Input: part model. Units: mm. Frame: model coordinates. A direction names the side the tool comes from. Coordinates: 2 decimals unless noted, no trailing zeros. Write each loop counter-clockwise with the first axis right and the second up, starting at its lowest first coordinate (ties: lowest second). Pieces come first, ordered by that corner, then holes. Notation, with made-up numbers: (23, -10.5) -> (70, -10.5) arc R14 cw to (70, -1.5) -> close; hole circle Ø1 at (-0.5, 84). An arc over 180 degrees is marked (long way). Use one line per item in the form item = value. Start each with the question number.
(1) First-contact query: pin 1 (5.5 mm diameter, centred on x = 8.31, z = 83.82, fed in from +Y); pin 2 (1.2 mm diameter, centred on x = -1, y = -1, fed in from +Z); pin 3 (1.9 mm diameter, centred on y = 1, z = 79, fed in from +X); pin 4 (2 mm diameter, centred on y = -1, z = 7.5, fed in from +X). Flat tips, straight axial feed; report the tip coordinate or a pass-through.
(2) Cut plane A-A on z = 0. Return the cut outline in (x, y) (3 decimals).
(3) Cut plane C-C on y = 2. Return the cut outline in (x, z) (3 decimals), plus the area to 3 significant figures.
(4) Ray query, line 1 along X through (y, z) = (1.25, 83.82); line 2 along X through (y, z) = (0, 0); line 3 along Z through (x, y) = (60, 1.75). Return the intervals inside material, ascending.
(5) Cut plane D-D on x = -28.5. Return the cut outline in (y, z) (3 decimals).
(6) Set-up query: faces 5 (the face through (-12.7, 0, 79)), 6 (the face through (12.7, 0, 79)), 7 (the face through (0, -2, 77.47)). Return all of +Z, -Z, +X, -X, +Y, -Y with unobstructed straight access to the full face (end or side cutting, diameter ignored); none if empty.
(7) Cut plane B-B on x = 0. Return the cut outline in (y, z) (3 decimals), plus the area to 3 significant figures.
(8) Pull-direction query (Z, two-part tool) for faces 1 (the face through (8.45, 0.04, 80.65)), 2 (the face through (20.6, -0.044, 65.413)), 3 (the face through (0.09, 0.89, 83.27)), 4 (the face through (0.1, 1.5, 88.9)); classes: released by +Z, released by -Z, zero draft, split by the parting line, or undercut.
```python
from build123d import *

# Parameters (mm, degrees)
SKETCH1_R                   = 76.2
SKETCH1_R_2                 = 68.58
BOSS_EXTRUDE1_DEPTH         = 3.175
BOSS_EXTRUDE2_DEPTH         = 6.35
FILLET1_R                   = 6.35
CUT_EXTRUDE1_DEPTH          = 11.43
F_3_8_0_25_DIAMETER_HOLE2_D = 6.35


with BuildPart() as part:
    # Sketch1 → Boss-Extrude1 (new, symmetric)
    with BuildSketch(Plane(origin=(0, 0, 0), x_dir=(1, 0, 0), z_dir=(0, 1, 0))):
        with Locations(Location((0, 0, 0), (0, 0, 270))):
            Circle(SKETCH1_R)
        with Locations(Location((0, 0, 0), (0, 0, 270))):
            Circle(SKETCH1_R_2, mode=Mode.SUBTRACT)
    extrude(amount=BOSS_EXTRUDE1_DEPTH, both=True)

    # Sketch2 → Boss-Extrude2 (add)
    with BuildSketch(Plane(origin=(0, 3.175, 0), x_dir=(1, 0, 0), z_dir=(0, 1, 0))):
        with BuildLine():
            Line((-12.7, -88.9), (-12.7, -75.134213245))
            ThreePointArc((-12.7, -75.134213245), (0, -76.2), (12.7, -75.134213245))
            Line((12.7, -75.134213245), (12.7, -88.9))
            Line((12.7, -88.9), (-12.7, -88.9))
        make_face()
    extrude(amount=-BOSS_EXTRUDE2_DEPTH)

    # Fillet1
    fillet1_edges = [part.edges().sort_by_distance(p)[0] for p in [
        (12.7, 0, 88.9),
        (-12.7, 0, 88.9),
    ]]
    fillet(fillet1_edges, radius=FILLET1_R)

    # Sketch3 → Cut-Extrude1 (cut)
    with BuildSketch(Plane.XY.offset(88.9)):
        with BuildLine():
            Line((-4.064, -3.175), (4.064, -3.175))
            ThreePointArc((4.064, -3.175), (0, 0.889), (-4.064, -3.175))
        make_face()
    extrude(amount=-CUT_EXTRUDE1_DEPTH, mode=Mode.SUBTRACT)

    # 3/8 (0.25) Diameter Hole2 (through all)
    with Locations(Plane(origin=(-8.3058, -3.175, 83.82), x_dir=(0, 0, -1), z_dir=(0, -1, 0))):
        with Locations((0, 0), (0, 16.6116)):
            Hole(F_3_8_0_25_DIAMETER_HOLE2_D / 2)


solid = part.part
```
Values:
q1.pin_1 = through
q1.pin_2 = 77.47
q1.pin_3 = 12.7
q1.pin_4 = 75.92
q2.outline = (-76.2, -3.175) -> (-68.58, -3.175) -> (-68.58, 3.175) -> (-76.2, 3.175) -> close; (68.58, -3.175) -> (76.2, -3.175) -> (76.2, 3.175) -> (68.58, 3.175) -> close
q3.outline = (-12.7, 75.134) arc R76.2 ccw (long way) to (12.7, 75.134) -> (12.7, 82.55) arc R6.35 ccw to (6.35, 88.9) -> (-6.35, 88.9) arc R6.35 ccw to (-12.7, 82.55) -> close; hole circle Ø137.16 at (0, 0); hole circle Ø6.35 at (-8.306, 83.82); hole circle Ø6.35 at (8.306, 83.82)
q3.area = 3,720 mm2
q4.line_1 = -12.57 to -11.48, -5.13 to 5.13, 11.48 to 12.57
q4.line_2 = -76.2 to -68.58, 68.58 to 76.2
q4.line_3 = -46.97 to -33.21, 33.21 to 46.97
q5.outline = (-3.175, -70.67) -> (3.175, -70.67) -> (3.175, -62.378) -> (-3.175, -62.378) -> close; (-3.175, 62.378) -> (3.175, 62.378) -> (3.175, 70.67) -> (-3.175, 70.67) -> close
q6.face_5 = +Z, -X, +Y, -Y
q6.face_6 = +Z, +X, +Y, -Y
q6.face_7 = +Z, -Y
q7.outline = (-3.175, -76.2) -> (3.175, -76.2) -> (3.175, -68.58) -> (-3.175, -68.58) -> close; (-3.175, 68.58) -> (3.175, 68.58) -> (3.175, 88.9) -> (0.889, 88.9) -> (0.889, 77.47) -> (-3.175, 77.47) -> close
q7.area = 131 mm2
q8.face_1 = undercut
q8.face_2 = undercut
q8.face_3 = zero draft
q8.face_4 = released by +Z
